Can you work these out from the model? Positions are in its coordinate system, mm. Round coordinates to 2 decimals unless told otherwise and drop trailing zeros. Order: outer loops, then holes, each group sorted by start corner. A loop starts at its lowest first (then second) coordinate and runs counter-clockwise, first axis right, second up. Notation, with made-up numbers: (31.25, 70) -> (80.25, 70) arc R18 ccw to (80.25, 82) -> close; hole circle Ø3 at (33, -20.5). An arc over 180 degrees is marked (long way). One line per item, written item: value.
```python
from build123d import *

# Parameters (mm, degrees)
F0_W     = 69.2285113037
F0_H     = 93.6287268996
F2_DEPTH = 76.2
F3_D     = 63.5
F3_DEPTH = 63.5
F3_TIP   = 19.0773246541


with BuildPart() as f2:
    # F0 (on Front) → F2 (new body)
    with BuildSketch(Plane.XZ):
        with Locations((1.5604775399, 6.6675022244)):
            Rectangle(F0_W, F0_H)
    extrude(amount=F2_DEPTH)

    # F3
    with Locations(Plane(origin=(0, 0, 0), x_dir=(1, 0, 0), z_dir=(0, 1, 0))):
        with Locations((0, -20.853670314)):
            Hole(F3_D / 2, depth=F3_DEPTH)
            with Locations((0, 0, -(F3_DEPTH + F3_TIP / 2))):  # 118° drill point
                Cone(0, F3_D / 2, F3_TIP, mode=Mode.SUBTRACT)


solid = f2.part
```
Q1. I want a section at A-A on x = 0. List the corners of the cut face in (y, z) for me.
Answers below:
outline: (-76.2, -40.15) -> (0, -40.15) -> (0, -10.9) -> (-63.5, -10.9) -> (-76.2, 10.24) -> close; (-76.2, 31.47) -> (-63.5, 52.6) -> (0, 52.6) -> (0, 53.48) -> (-76.2, 53.48) -> close
Q2. Please list where these lines run through material, in increasing order: line 1 along Z through (x, y) = (0, -32.5); line 2 along X through (y, z) = (-46, 18); line 3 along X through (y, z) = (-67, 28).
Answers below:
line 1: -40.15 to -10.9, 52.6 to 53.48
line 2: -33.05 to -31.62, 31.62 to 36.17
line 3: -33.05 to -24.92, 24.92 to 36.17
Q3. Will this pin go through, and if not, where does the flat tip stop? pin 1 Ø5 at (x, z) = (24, 11.5) entering from +Y.
Answers below:
pin 1: y = -65.6
Q4. I want a section at B-B on y = -29.5. List the corners of the cut face in (x, z) for me, plus the area to 3 significant figures.
Answers below:
outline: (-33.05, -40.15) -> (36.17, -40.15) -> (36.17, 53.48) -> (-33.05, 53.48) -> close; hole circle Ø63.5 at (0, 20.85)
area: 3,310 mm^2
Q5. We'd pull the mould along Z, two halves only. Please class faces 1 (the face through (-1.554, -75.406, 9.019)), 2 (the face through (-33.054, -38, 6)), 3 (the face through (1, -38, -40.147)), 4 (the face through (4.133, -32.195, -10.626)): released by +Z, released by -Z, zero draft, split by the parting line, or undercut.
Answers below:
face 1: undercut
face 2: zero draft
face 3: released by -Z
face 4: undercut
